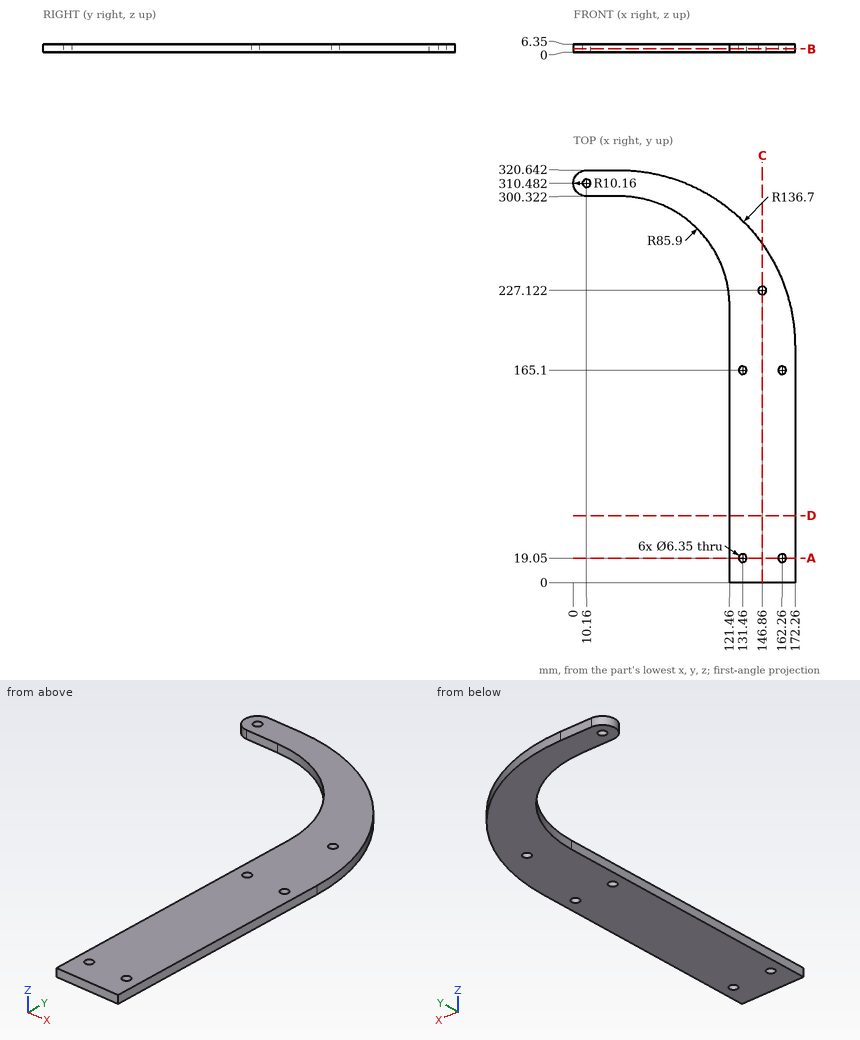
Geometry: see drawing. Coordinates: mm, zero at the bounding-box minimum. Give positions to 0.01 mm unless a question says otherwise; leave off trailing zeros. Order: outer loops, then holes, each group sorted by start corner. A loop starts at its lowest first (then second) coordinate and runs counter-clockwise, first axis right, second up.
1. Pin query (flat end, axial travel): pin 1 Ø2 at (x, y) = (123.5, 168.5) entering from -Z; pin 2 Ø1.5 at (x, z) = (128, 5.5) entering from +Y; pin 3 Ø1 at (x, z) = (137.5, 1) entering from +Y; pin 4 Ø3 at (y, z) = (125.5, 4) entering from -X. Return the tip coordinate at first contact, or that it passes through.
Computed:
pin 1: stops at z = 0
pin 2: stops at y = 285.33
pin 3: stops at y = 275.58
pin 4: stops at x = 121.46
2. Cut plane A-A (y = 19.05). Return loops of the section in (x, z) (3 decimals), and give its area (3 significant figures).
Computed:
outline: (121.46, 0) - (128.285, 0) - (128.285, 6.35) - (121.46, 6.35) - close; (134.635, 0) - (159.085, 0) - (159.085, 6.35) - (134.635, 6.35) - close; (165.435, 0) - (172.26, 0) - (172.26, 6.35) - (165.435, 6.35) - close
area: 242 mm2
3. Line query: probe 1 along X at (y, z) = (165.1, 5.25) (3 decimals); probe 2 along Y at (x, z) = (131.46, 3.25) (1 decimal); probe 3 along X at (y, z) = (164, 3). Output: solid intervals per line, ascending.
Computed:
probe 1: x = 121.46 to 128.285, 134.635 to 159.085, 165.435 to 172.26
probe 2: y = 0 to 15.9, 22.2 to 161.9, 168.3 to 281.4
probe 3: x = 121.46 to 128.48, 134.44 to 159.28, 165.24 to 172.26
4. Cut plane B-B (z = 2.5). State how many separate pieces and enclosed holes the cut face has, and give its area (3 significant figures).
Computed:
separate pieces: 1
enclosed holes: 6
area: 16,100 mm2
5. Cut plane D-D (y = 52). Return loops of the section in (x, z), and give its area (3 significant figures).
Computed:
outline: (121.46, 0) - (172.26, 0) - (172.26, 6.35) - (121.46, 6.35) - close
area: 323 mm2
6. Cut plane C-C (x = 146.86). Return loops of the section in (y, z).
Computed:
outline: (0, 0) - (223.95, 0) - (223.95, 6.35) - (0, 6.35) - close; (230.3, 0) - (263.31, 0) - (263.31, 6.35) - (230.3, 6.35) - close
